Geometry: see drawing. Coordinates: mm, zero at the bounding-box minimum. Coordinates: 2 decimals unless noted, no trailing zeros. Loops run counter-clockwise (first coordinate to the right, second up) from the corner with the lowest first, then second, coordinate; pieces in that order, holes last. Notation, with made-up numbers: (5, -16) -> (24, -16) arc R13 cw to (24, -12) -> close; hole circle Ø3 at (61, 61.25). An arc over 180 degrees is marked (long way). Put each result on its own line as item: value. Start each with the question number.
1) Material intervals for L1, parallel to Y at x = 26, z = 47.5; L2, parallel to Z at x = 31.5, y = 33.5; L3, parallel to X at y = 45, z = 48, sorted ascending.
2) Pull-direction query (X, two-part tool) for the marked faces 1, 2 and 3; classes: pulls with the +X half, pulls with the -X half, needs draft (parallel to the pull), parting line crosses it, or undercut.
3) Cut plane A-A (y = 6.5). Return the cut outline in (x, z), plus the area to 3 significant figures.
4) Contact query for a flat-ended pin moving along its axis: P1, Ø1, axis at x = 28.5, y = 31, coming from the +Z side. Output: stop coordinate, or through.
5) Cut plane B-B (x = 36.5). Return the cut outline in (y, z), plus the area to 3 significant figures.
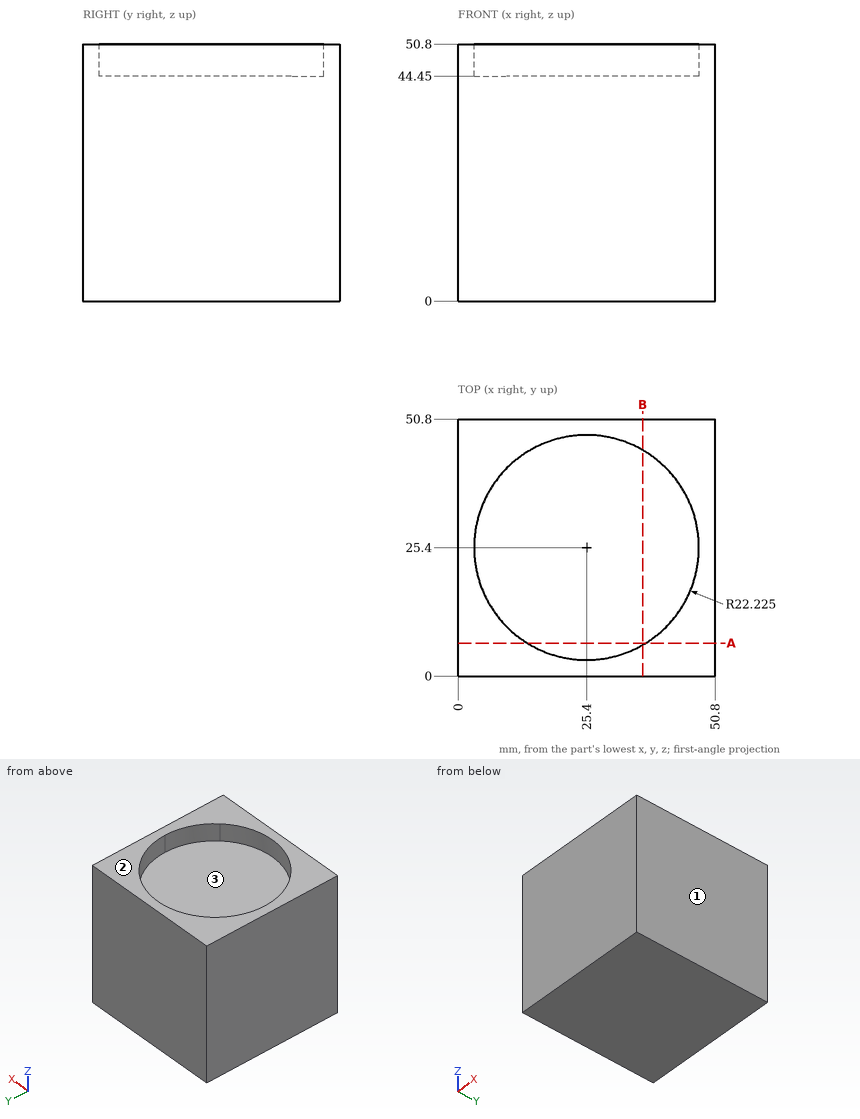
Results found:
1. L1: y = 0 to 3.18, 47.62 to 50.8
1. L2: z = 0 to 44.45
1. L3: x = 0 to 14.92, 35.88 to 50.8
2. face 1: pulls with the +X half
2. face 2: needs draft
2. face 3: undercut
3. outline: (0, 0) -> (50.8, 0) -> (50.8, 50.8) -> (37.09, 50.8) -> (37.09, 44.45) -> (13.71, 44.45) -> (13.71, 50.8) -> (0, 50.8) -> close
3. area: 2,430 mm2
4. P1: stops at z = 44.45
5. outline: (0, 0) -> (50.8, 0) -> (50.8, 50.8) -> (44.65, 50.8) -> (44.65, 44.45) -> (6.15, 44.45) -> (6.15, 50.8) -> (0, 50.8) -> close
5. area: 2,340 mm2
